from build123d import *

# Parameters (mm, degrees)
BOSS_EXTRUDE1_DEPTH = 3
CUT_EXTRUDE3_DEPTH  = 516.692890771
SKETCH4_R           = 1.64
CUT_EXTRUDE2_DEPTH  = 516.692890771


with BuildPart() as part:
    # Sketch1 → Boss-Extrude1 (new body)
    with BuildSketch(Plane.XY):
        Polygon((-398.2841, 298.0765), (-386.271234014, 299.794262601), (-339.587365996, 299.794262601), (-339.587365996, 281.358737399), (-386.271234014, 281.358737399), (-398.2841, 283.0765), (-419.587365996, 283.0765), (-419.587365996, 298.0765), align=None)
    extrude(amount=BOSS_EXTRUDE1_DEPTH)

    # Sketch5 → Cut-Extrude3 (cut, through all)
    with BuildSketch(Plane(origin=(0, 0, 0), x_dir=(-1, 0, 0), z_dir=(0, 0, -1))):
        with BuildLine():
            Line((403.321087066, 293.299611149), (403.321087066, 287.899611149))
            ThreePointArc((403.321087066, 287.899611149), (407.635649248, 290.599611149), (403.321087066, 293.299611149))
        make_face()
    extrude(amount=-CUT_EXTRUDE3_DEPTH, mode=Mode.SUBTRACT)

    # Sketch4 → Cut-Extrude2 (cut, through all)
    with BuildSketch(Plane(origin=(0, 0, 0), x_dir=(-1, 0, 0), z_dir=(0, 0, -1))):
        with Locations((355.605649248, 290.599611149)):
            Circle(SKETCH4_R)
    extrude(amount=-CUT_EXTRUDE2_DEPTH, mode=Mode.SUBTRACT)


solid = part.part
CAD build for the part. Positions are in the model's coordinates, mm. A direction names the side the tool comes from. Round coordinates to 2 decimals unless told otherwise and drop trailing zeros. Write each loop counter-clockwise with the first axis right and the second up, starting at its lowest first coordinate (ties: lowest second). Pieces come first, ordered by that corner, then holes. Notation, with made-up numbers: M -4.5,11 L 32.5,11 A16 cw 32.5,34 Z; hole C 33,38 d3. An arc over 180 degrees is marked long. Put each result on its own line as item: value. Start each with the question number.
1) Saw through at B-B, the plane y = 289.75. Write the cut outline in (x, z).
2) Pin check, flat tip, straight feed: pin 1 Ø1.5 at (x, z) = (-407, 1) entering from -Y. Stop position of the tip, or through.
3) Pull direction Y, two halves, no side cores. Call faces 3 (the cylindrical face through (-355.392, 292.226, 1.479)), 4 (the flat face through (-409, 298.076, 1)), 5 (the flat face through (-409, 283.076, 1)): pulls with the +Y half, pulls with the -Y half, needs draft (parallel to the pull), parting line crosses it, or undercut.
4) Drill centre lines: probe 1 along X at (y, z) = (291, 0.95); probe 2 along X at (y, z) = (292, 0.4); probe 3 along Y at (x, z) = (-404.5, 1.9). Where is each one in solid material? Low to high. Write a range as [from, to].
5) Saw through at C-C, the plane z = 2.1. Write the cut outline in (x, y).
6) Saw through at D-D, the plane x = -391. Write the cut outline in (y, z).
7) 3-axis set-ups, long thin cutter, end or side, ignore diameter. For faces 1 (the flat face through (-403.321, 291, 1)), 2 (the flat face through (-379, 291, 0)): which of +Z, -Z, +X, -X, +Y, -Y reach the whole face in a straight line?
8) Saw through at A-A, the plane x = -356. Write the cut outline in (y, z), and give its area (3 significant figures).
Resolved:
1. outline: M -419.59,0 L -407.51,0 L -407.51,3 L -419.59,3 Z; M -403.32,0 L -357.01,0 L -357.01,3 L -403.32,3 Z; M -354.2,0 L -339.59,0 L -339.59,3 L -354.2,3 Z
2. pin 1: y = 283.08
3. face 3: undercut
3. face 4: pulls with the +Y half
3. face 5: pulls with the -Y half
4. probe 1: [-419.59, -407.61], [-403.32, -357.2], [-354.02, -339.59]
4. probe 2: [-419.59, -407.29], [-403.32, -356.46], [-354.75, -339.59]
4. probe 3: [283.08, 287.6], [293.6, 298.08]
5. outline: M -419.59,283.08 L -398.28,283.08 L -386.27,281.36 L -339.59,281.36 L -339.59,299.79 L -386.27,299.79 L -398.28,298.08 L -419.59,298.08 Z; hole M -403.32,287.9 L -403.32,293.3 A3 ccw long Z; hole C -355.61,290.6 d3.28
6. outline: M 282.03,0 L 299.12,0 L 299.12,3 L 282.03,3 Z
7. face 1: +Z, -Z
7. face 2: -Z, +X, -X, +Y, -Y
8. outline: M 281.36,0 L 289.01,0 L 289.01,3 L 281.36,3 Z; M 292.19,0 L 299.79,0 L 299.79,3 L 292.19,3 Z
8. area: 45.8 mm²
